Build history of the part. All positions in model axes, mm. A direction names the side the tool comes from. Coordinates: 2 decimals unless noted, no trailing zeros. Loops run counter-clockwise (first coordinate to the right, second up) from the corner with the lowest first, then second, coordinate; pieces in that order, holes last. Notation, with made-up numbers: (47, 27.5) - (97, 27.5) arc R21 ccw to (97, 61.5) - close; hole circle Ø8 at (79, 47). An arc over 180 degrees is marked (long way). One line per item, written item: value.
```python
from build123d import *

# Parameters (mm, degrees)
F0_W     = 210
F0_H     = 200
F1_DEPTH = 400
F2_W     = 920
F2_H     = 200
F3_DEPTH = 100
F4_W     = 60
F4_H     = 200
F5_DEPTH = 100


with BuildPart() as f1:
    # F0 (on Top) → F1 (new body)
    with BuildSketch(Plane.XY):
        with Locations((-420, -100)):
            Rectangle(F0_W, F0_H)
        with Locations((420, -100)):
            Rectangle(F0_W, F0_H)
    extrude(amount=F1_DEPTH)

    # F2 (on face) → F3 (join)
    with BuildSketch(Plane.XY.offset(400)):
        with Locations((0, -100)):
            Rectangle(F2_W, F2_H)
    extrude(amount=F3_DEPTH)

    # F4 (on face) → F5 (join)
    with BuildSketch(Plane.XY.offset(400)):
        with Locations((-495, -100)):
            Rectangle(F4_W, F4_H)
        with Locations((495, -100)):
            Rectangle(F4_W, F4_H)
    extrude(amount=F5_DEPTH)


solid = f1.part
```
Item 1: Cut at A-A, the plane z = 40.5. Write the cut outline in (x, y), then the cut area to 3 significant figures.
Check result:
outline: (-525, -200) - (-315, -200) - (-315, 0) - (-525, 0) - close; (315, -200) - (525, -200) - (525, 0) - (315, 0) - close
area: 84,000 mm^2
Item 2: Drop flat-ended pins along their axis: P1, Ø1.5, axis at x = 462, y = -119.5, coming from the +Z side; P2, Ø1.5, axis at x = 34.5, y = -21.5, coming from the -Z side. Give the stop position or say it passes through.
Check result:
P1: stops at z = 400
P2: stops at z = 400
Item 3: Cut at C-C, the plane x = 98. Write the cut outline in (y, z), then the cut area to 3 significant figures.
Check result:
outline: (-200, 400) - (0, 400) - (0, 500) - (-200, 500) - close
area: 20,000 mm^2
Item 4: Tool access for faces 1 (the face through (-465, -101, 449)), 2 (the face through (-421, -99, 0)), 3 (the face through (315, -101, 197)): list every direction of +Z, -Z, +X, -X, +Y, -Y with a clear straight run to the whole face (end or side of a thin tool).
Check result:
face 1: +Z, +Y, -Y
face 2: -Z, +X, -X, +Y, -Y
face 3: -Z, +Y, -Y
Item 5: Probe probe 1 along X at (y, z) = (-70, 125.5); probe 2 along Z at (x, y) = (-122.5, -166). List the from-to ranges inside material, lowest first. Write a range as from..to.
Check result:
probe 1: x = -525..-315, 315..525
probe 2: z = 400..500
Item 6: Cut at B-B, the plane y = -77.5. Write the cut outline in (x, z), then the cut area to 3 significant figures.
Check result:
outline: (-525, 0) - (-315, 0) - (-315, 400) - (315, 400) - (315, 0) - (525, 0) - (525, 500) - (465, 500) - (465, 400) - (460, 400) - (460, 500) - (-460, 500) - (-460, 400) - (-465, 400) - (-465, 500) - (-525, 500) - close
area: 272,000 mm^2
